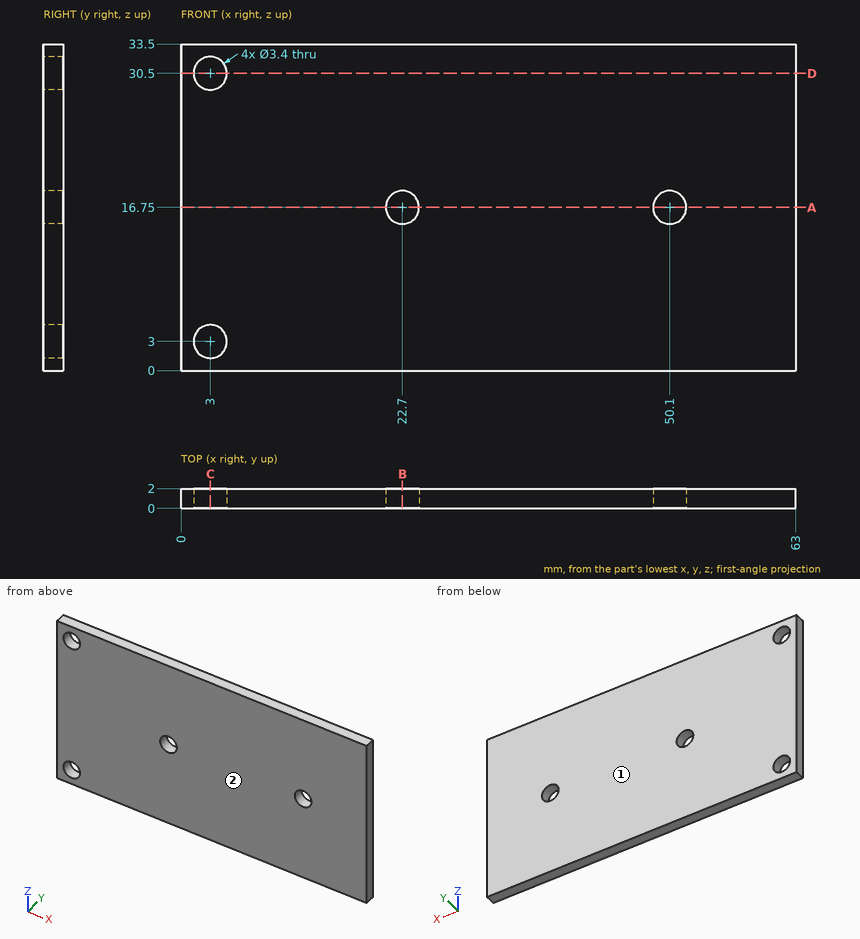
Study the drawing (mm; zero at the part's minimum x, y, z) and answer. Give positions to 0.01 mm unless a question says otherwise; leave off trailing zeros. Order: outer loops, then holes, each group sorted by start corner. A loop starts at its lowest first (then second) coordinate and runs counter-clockwise, first axis right, second up. Notation, with made-up numbers: (71, 7) - (93, 7) arc R8 ccw to (93, 20) - close; hole circle Ø3 at (7, 45). An arc over 180 degrees is marked (long way). Use one line per item in the form item = value. Start each with the question number.
(1) A cutting plane is placed at B-B, the plane x = 22.7. Write down the section's boundary in (y, z), then the cut area to 3 significant figures.
(2) Consider line 1 (X direction, y = 1.3, z = 16.75); line 2 (Z direction, x = 3, y = 1.5); line 3 (X direction, y = 1.1, z = 17.5). Determine where each line is inside the solid, lowest interval first. Write a range as from..to.
(3) A flat-ended cylindrical pin translates along its axis: pin 1 Ø4.5 at (x, z) = (3, 30.5) entering from +Y. Find the tip coordinate at first contact, or state that the pin passes through.
(4) A cutting plane is placed at D-D, the plane z = 30.5. Write down the section's boundary in (x, y), then the cut area to 3 significant figures.
(5) The mould has two halves that part along Y. Classify the marked faces 1 and 2: released by +Y, released by -Y, zero draft, split by the parting line, or undercut.
(6) A cutting plane is placed at C-C, the plane x = 3. Write down the section's boundary in (y, z), then the cut area to 3 significant figures.
(7) A cutting plane is placed at A-A, the plane z = 16.75. Write down the section's boundary in (x, y), then the cut area to 3 significant figures.
Ans:
q1.outline = (0, 0) - (2, 0) - (2, 15.05) - (0, 15.05) - close; (0, 18.45) - (2, 18.45) - (2, 33.5) - (0, 33.5) - close
q1.area = 60.2 mm^2
q2.line_1 = 0..21, 24.4..48.4, 51.8..63
q2.line_2 = 0..1.3, 4.7..28.8, 32.2..33.5
q2.line_3 = 0..21.17, 24.23..48.57, 51.63..63
q3.pin_1 = 2
q4.outline = (0, 0) - (1.3, 0) - (1.3, 2) - (0, 2) - close; (4.7, 0) - (63, 0) - (63, 2) - (4.7, 2) - close
q4.area = 119 mm^2
q5.face_1 = released by +Y
q5.face_2 = released by -Y
q6.outline = (0, 0) - (2, 0) - (2, 1.3) - (0, 1.3) - close; (0, 4.7) - (2, 4.7) - (2, 28.8) - (0, 28.8) - close; (0, 32.2) - (2, 32.2) - (2, 33.5) - (0, 33.5) - close
q6.area = 53.4 mm^2
q7.outline = (0, 0) - (21, 0) - (21, 2) - (0, 2) - close; (24.4, 0) - (48.4, 0) - (48.4, 2) - (24.4, 2) - close; (51.8, 0) - (63, 0) - (63, 2) - (51.8, 2) - close
q7.area = 112 mm^2
